Autodesk Inventor part; units mm, degrees
ref_plane "YZ Plane" through (0, 0, 0) normal (1, 0, 0) x (0, 1, 0)
ref_plane "XZ Plane" through (0, 0, 0) normal (0, 1, 0) x (-1, 0, 0)
ref_plane "XY Plane" through (0, 0, 0) normal (0, 0, 1) x (1, 0, 0)
sketch "スケッチ1" plane through (0, 0, 0) normal (0, 0, 1) x (1, 0, 0)
  line L0 (-170.6512, -31.4118) -> (202.8656, -31.4118) construction
  circle A0 centre (-14, -17.4118) radius 14 construction
  circle A1 centre (14, -17.4118) radius 14 construction
  circle A2 centre (-28.0204, 0.0121) radius 20.05 construction
  circle A3 centre (-28.0204, 0.0121) radius 5.05 construction
  circle A4 centre (8.8763, 3.8907) radius 32.05 construction
  circle A5 centre (8.8763, 3.8907) radius 10.1 construction
  circle A6 centre (54.047, 13.5882) radius 36.1 construction
  line L1 (-170.915, -81.4118) -> (490.0044, -81.4118)
  circle A7 centre (-28.0204, 0.0121) radius 22.342 construction
  circle A8 centre (-39.4931, 19.1835) radius 14 construction
  circle A9 centre (-49.0547, 7.5438) radius 14 construction
  circle A10 centre (-49.0547, -7.5196) radius 14 construction
  circle A11 centre (-39.4931, -19.1593) radius 14 construction
  circle A12 centre (8.8763, 3.8907) radius 33.05 construction
  circle A13 centre (54.047, 13.5882) radius 38.1 construction
  line L2 (-11.5565, -29.1593) -> (4.2969, -29.1593) construction
  line L3 (-67.2952, 44.8622) -> (-67.2952, -57.3934) construction
  line L4 (-149.4523, -1.6098) -> (-132.6633, -31.6026)
  line L5 (-132.7701, -31.4118) -> (-132.7701, 74.0456)
  circle A14 centre (-11.4931, -19.1593) radius 14 construction
  line L6 (-197.2268, -33.1593) -> (179.6604, -33.1593) construction
  circle A15 centre (54.047, 13.5882) radius 4.025
  circle A16 centre (54.047, 13.5882) radius 6
  circle A17 centre (-39.4931, 19.1835) radius 5
  circle A18 centre (-49.0547, 7.5438) radius 5
  circle A19 centre (-49.0547, -7.5196) radius 5
  circle A20 centre (-39.4931, -19.1593) radius 5
  circle A21 centre (-39.4931, 19.1835) radius 8 construction
  circle A22 centre (-49.0547, 7.5438) radius 8 construction
  circle A23 centre (-49.0547, -7.5196) radius 8 construction
  circle A24 centre (-39.4931, -19.1593) radius 8 construction
  circle A25 centre (-28.0204, 0.0121) radius 4.5
  circle A26 centre (8.8763, 3.8907) radius 7.5
  line L7 (-17.5497, 32.3149) -> (-46.3578, 15.0755) construction
  line L8 (-46.3578, 15.0755) -> (-51.7515, 0.0121) construction
  line L9 (-51.7515, 0.0121) -> (-46.3578, -15.0513) construction
  line L10 (-46.3578, -15.0513) -> (-37.9391, -20.0892) construction
  circle A27 centre (-32.6283, 23.2915) radius 1.3
  circle A28 centre (-46.3578, 15.0755) radius 1.3
  circle A29 centre (-51.7515, 0.0121) radius 1.3
  circle A30 centre (-46.3578, -15.0513) radius 1.3
  circle A31 centre (-32.6283, -23.2673) radius 1.3
  line L11 (-67.2952, 23.1796) -> (-67.2952, -18.1327)
  arc A32 (79.2003, -37.212) -> (87.3507, -31.2711) centre (80.4159, -30.3183) ccw
  arc A33 (8.1864, 50.8943) -> (0.9804, 51.9708) centre (3.7003, 45.5208) ccw
  line L12 (-52.2685, -33.1593) -> (56.2168, -33.1593)
  line L13 (56.2168, -33.1593) -> (79.2003, -37.212)
  arc A34 (92.7831, 8.2659) -> (29.742, 44.2162) centre (54.047, 13.5882) ccw
  line L14 (87.3507, -31.2711) -> (92.7831, 8.2659)
  line L15 (0.9804, 51.9708) -> (-67.2952, 23.1796)
  circle A35 centre (34.0114, -24.0061) radius 4.5 construction
  circle A36 centre (34.0114, -24.0061) radius 1.5
  circle A37 centre (-21.4477, 26.0369) radius 4.5 construction
  circle A38 centre (-21.4477, 26.0369) radius 1.5
  circle A39 centre (-56.0504, 23.0377) radius 1.5
  circle A40 centre (-56.0504, 23.0377) radius 3 construction
  circle A41 centre (-56.0504, 23.0377) radius 4.5 construction
  circle A42 centre (-64.2952, 0.0121) radius 1.5
  circle A43 centre (-64.2952, 0.0121) radius 3 construction
  circle A44 centre (-64.2952, 0.0121) radius 4.3311 construction
  line L16 (54.047, 13.5882) -> (103.0278, 23.6322)
  line L17 (103.0278, 23.6322) -> (59.4403, 12.4461)
  line L18 (59.4403, 12.4461) -> (30.7326, 32.4678)
  line L19 (30.7326, 32.4678) -> (54.047, 13.5882)
  line L20 (103.0278, 23.6322) -> (519.5307, 130.5215)
  line L21 (-183.2789, 162.2213) -> (-183.2789, -125.2315)
  line L22 (516.7211, 155.5913) -> (516.7211, -155.5644)
  circle A45 centre (103.0278, 23.6322) radius 7.25
  arc A46 (101.805, 33.809) -> (106.8568, 14.1242) centre (103.0278, 23.6322) ccw
  line L23 (141.7723, 33.5754) -> (440.8907, 56.5571) construction
  line L24 (241.9124, 41.2693) -> (202.3713, 99.0317) construction
  circle A47 centre (3.7003, 45.5208) radius 4
  circle A48 centre (127.2431, 29.8467) radius 2
  circle A49 centre (141.7723, 33.5754) radius 2
  arc A50 (143.6401, 28.9373) -> (141.1758, 38.5397) centre (141.7723, 33.5754) ccw
  line L25 (143.6401, 28.9373) -> (106.8568, 14.1242)
  line L26 (141.1758, 38.5397) -> (101.805, 33.809)
  circle A51 centre (30.7326, 32.4678) radius 2
  circle A52 centre (-16.1798, -24.0771) radius 4.5 construction
  circle A53 centre (-16.1798, -24.0771) radius 1.5
  line L27 (-67.2952, -18.1327) -> (-52.2685, -33.1593)
  circle A54 centre (-56.0504, -23.0135) radius 1.5
  circle A55 centre (-56.0504, -23.0135) radius 3 construction
  circle A56 centre (30.7326, 32.4678) radius 4
  arc A57 (55.034, 16.9462) -> (53.2318, 10.1845) centre (54.047, 13.5882) ccw
  line L28 (99.9171, 22.9943) -> (104.0308, 26.6451) construction
  line L29 (104.0308, 26.6451) -> (105.1356, 21.2572) construction
  line L30 (105.1356, 21.2572) -> (99.9171, 22.9943) construction
  circle A58 centre (105.1356, 21.2572) radius 1.5
  circle A59 centre (104.0308, 26.6451) radius 1.5
  circle A60 centre (99.9171, 22.9943) radius 1.5
  circle A61 centre (103.0278, 23.6322) radius 6
  arc A62 (106.7324, 15.9819) -> (96.5933, 29.1862) centre (103.0278, 23.6322) ccw
  arc A63 (55.034, 16.9462) -> (96.5933, 29.1862) centre (66.3134, 55.3229) ccw
  arc A64 (53.2318, 10.1845) -> (106.7324, 15.9819) centre (71.8656, 87.9841) ccw
  circle A65 centre (54.047, 13.5882) radius 8.5
  line L31 (101.3203, 31.9589) -> (52.3395, 21.9149)
  line L32 (55.7545, 5.2615) -> (104.7353, 15.3054)
  circle A66 centre (12.7384, 41.2415) radius 3 construction
  circle A67 centre (12.7384, 41.2415) radius 4.5 construction
  circle A68 centre (12.7384, 41.2415) radius 1.5
  circle A69 centre (80.4159, -30.3183) radius 4
  circle A70 centre (69.7531, -26.0108) radius 1.5
  circle A71 centre (69.7531, -26.0108) radius 4.5 construction
  circle A72 centre (-56.0504, -23.0135) radius 4.5 construction
  line L33 (8.1864, 50.8943) -> (15.9809, 44.3871)
  arc A73 (15.9809, 44.3871) -> (29.742, 44.2162) centre (22.9664, 52.7545) ccw
  circle A74 centre (-5.4761, 38.5895) radius 1.5
  circle A75 centre (-5.4761, 38.5895) radius 4.5 construction
  circle A76 centre (54.047, 13.5882) radius 50 construction
  circle A77 centre (3.7003, 45.5208) radius 2
  circle A78 centre (80.4159, -30.3183) radius 2
  circle A79 centre (54.047, 13.5882) radius 1.5
  point P0 (0, 0)
  point P1 (0, 0)
  point P2 (-49.0547, 7.5438)
  point P3 (-49.0547, -7.5196)
  dimension "d89" = 100
  dimension "d0" = 40.1
  dimension "d1" = 10.1
  dimension "d2" = 64.1
  dimension "d3" = 20.2
  dimension "d4" = 72.2
  dimension "d5" = 95
  dimension "d6" = 44.684
  dimension "d7" = 28
  dimension "d8" = 28
  dimension "d9" = 28
  dimension "d10" = 28
  dimension "d11" = 1
  dimension "d12" = 2
  dimension "d13" = 4
  dimension "d14" = 8.05
  dimension "d15" = 12
  dimension "d16" = 10
  dimension "d17" = 10
  dimension "d18" = 10
  dimension "d19" = 10
  dimension "d20" = 3
  dimension "d21" = 3
  dimension "d22" = 3
  dimension "d23" = 3
  dimension "d24" = 9
  dimension "d25" = 15
  dimension "d26" = 2.6
  dimension "d27" = 2.6
  dimension "d28" = 2.6
  dimension "d29" = 2.6
  dimension "d30" = 2.6
  dimension "d31" = 1
  dimension "d32" = 9
  dimension "d33" = 3
  dimension "d34" = 9
  dimension "d35" = 3
  dimension "d36" = 3
  dimension "d37" = 6
  dimension "d38" = 9
  dimension "d39" = 3
  dimension "d40" = 6
  dimension "d41" = 50
  dimension "d42" = 45
  dimension "d43" = 35
  dimension "d44" = 30
  dimension "d45" = 39
  dimension "d46" = 430
  dimension "d47" = 700
  dimension "d48" = 14.5
  dimension "d49" = 3
  dimension "d50" = 300
  dimension "d51" = 10
  dimension "d52" = 70
  dimension "d53" = 120
  dimension "d54" = 140
  dimension "d55" = 8
  dimension "d56" = 4
  dimension "d57" = 4
  dimension "d58" = 15
  dimension "d59" = 25
  dimension "d60" = 10
  dimension "d61" = 4
  dimension "d62" = 9
  dimension "d63" = 3
extrude "押し出し1" add sketch "スケッチ1" along normal blind 3 contours A15 L18 L16 | A15 L16 A16 L17 L18 | L16 L18 A57 A63 A15 | A15 A63 A16 L16 | L18 L17 A16 A64 A15 | A15 A64 A57 L19 A79 L16 L18 | L16 A79 L19 A57 L18 | L16 A65 L17 A16 | A16 A63 A65 L16 | A65 A63 L16 | L16 A63 L17 A65 | A16 L17 A65 A64 | A65 L17 A63 A34 L32 A64 | A63 A34 L16 | L16 A34 L17 A63 | L32 A34 A64 | L16 A46 L17 A34 | A34 A63 A46 L16 | A34 L32 A46 A64 | A34 L17 A46 L32 | A46 A63 A62 L20 A45 L16 | L16 A45 L17 A46 | A46 L17 A45 L20 A62 A64 | A45 L20 A61 L16 | L16 A61 L17 A45 | L17 A61 L20 A45 | A61 L20 L16 A60 | L16 A60 L17 A61 | L17 A60 L20 A61 | L16 L17 A60 picked at (101.9354, 23.3989)
properties part number "アーム駆動抑え" material "アルミニウム 2014-T4"
Geometry check sheet. Reference: the model listing, model coordinates, mm. Coordinates: 2 decimals unless noted, no trailing zeros. Order: outer loops, then holes, each group sorted by start corner. A loop starts at its lowest first (then second) coordinate and runs counter-clockwise, first axis right, second up. Notation, with made-up numbers: M 14,32.25 L 19,32.25 A20 cw 19,39.25 Z; hole C -4.75,44 d10. An arc over 180 degrees is marked long. Use CSV: the item, a comma, the result in double quotes.
Item 1: Mould release check, pull along Y, two halves, no side actions. Record for faces 1 (the cylindrical face through (105.46, 26.19, 1.48)), 2 (the cylindrical face through (80.866, 8.492, 1.479)), 3 (the flat face through (87, 18, 0)), 4 (the cylindrical face through (50.646, 14.414, 1.479)): pulls with the +Y half, pulls with the -Y half, needs draft (parallel to the pull), parting line crosses it, or undercut.
Returned:
face 1,"undercut"
face 2,"pulls with the -Y half"
face 3,"needs draft"
face 4,"parting line crosses it"
Item 2: Cross-section at D-D on x = 74. Record the cut outline in (y, z), then the cut area to 3 significant figures.
Returned:
outline,"M 8.01,0 L 16.07,0 L 16.07,3 L 8.01,3 Z"
area,"24.2 mm2"
Item 3: Cross-section at B-B on z = 1.1. Record the cut outline in (x, y), then the cut area to 3 significant figures.
Returned:
outline,"M 53.23,10.18 A80 ccw 106.73,15.98 A8.5 ccw long 96.59,29.19 A40 cw 55.03,16.95 A3.5 ccw long Z; hole C 54.05,13.59 d3; hole C 99.92,22.99 d3; hole C 104.03,26.65 d3; hole C 105.14,21.26 d3"
area,"627 mm2"
Item 4: Cross-section at C-C on x = 97.5. Record the cut outline in (y, z).
Returned:
outline,"M 12.2,0 L 30.09,0 L 30.09,3 L 12.2,3 Z"
Item 5: Gauge pin test, flat ends, axial feed: pin 1 Ø2.5 at (x, y) = (99.92, 22.99) entering from -Z; pin 2 Ø10 at (x, y) = (57, 20.5) entering from +Z. Record the tip position at first contact, or that the pin passes through.
Returned:
pin 1,"passes through"
pin 2,"stops at z = 3"
Item 6: Cross-section at A-A on y = 20.5. Record the cut outline in (x, z).
Returned:
outline,"M 85.99,0 L 103.84,0 L 103.84,3 L 85.99,3 Z; M 106.43,0 L 110.93,0 L 110.93,3 L 106.43,3 Z"
Item 7: Thickness scan on line 1 along X through (y, z) = (22.5, 1.4); line 2 along Y through (x, z) = (99.5, 1.05); line 3 along Y through (x, z) = (103.5, 2.5). Record the ranges inside material, lowest first.
Returned:
line 1,"x = 89.18 to 98.5, 101.33 to 104.3, 105.98 to 111.45"
line 2,"y = 12.91 to 21.55, 24.44 to 31.37"
line 3,"y = 14.5 to 25.24, 28.05 to 32.12"
